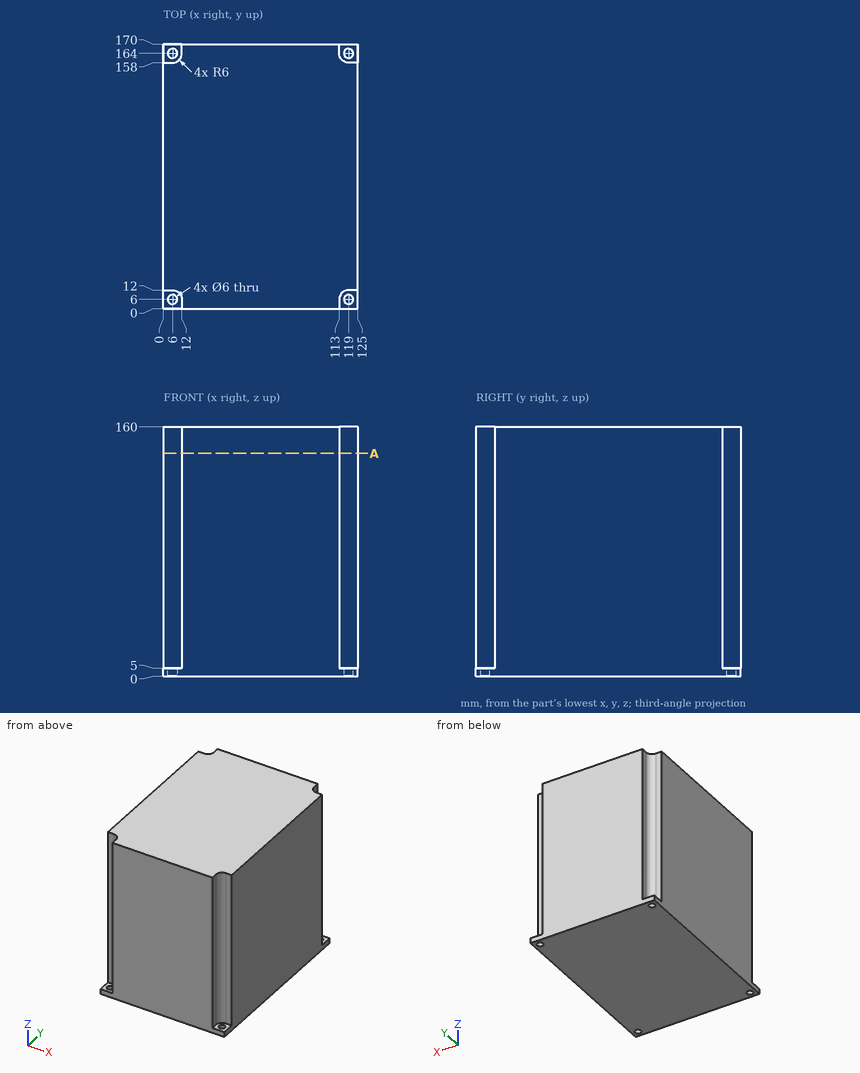
Geometry check sheet. Reference: drawing and pictorial views, mm from the part's lowest x, y, z. Give positions to 0.01 mm unless a question says otherwise; leave off trailing zeros. Write each loop counter-clockwise with the first axis right and the second up, starting at its lowest first coordinate (ties: lowest second). Pieces come first, ordered by that corner, then holes. Notation, with made-up numbers: M 11.25,70 L 45.25,70 A25 cw 45.25,98 Z; hole C 56.25,43.25 d10. An arc over 180 degrees is marked long. Answer as CSV lines item,"result". Start each with the question number.
Q1. Section check A-A, the plane z = 143. Record the cut outline in (x, y), then the cut area to 3 significant figures.
Q2. Go/stop test with flat-tipped pins: pin 1 (1.8 mm diameter, centred on y = 168, z = 118.5, fed in from -X); pin 2 (3 mm diameter, centred on x = 2.5, z = 54.5, fed in from -Y); pin 3 (1.8 mm diameter, centred on x = 121.5, z = 77.5, fed in from +Y); pin 4 (5 mm diameter, centred on x = 119, y = 164, fed in from -Z). Record where each tip stops, or that it passes through.
Q3. Material ranges on L1, parallel to Y at x = 119, z = 2; L2, parallel to X at y = 164, z = 3.95; L3, parallel to X at y = 8.5, z = 55, recorded low to high.
Geometry says:
1,outline,"M 0,12 L 6,12 A6 cw 12,6 L 12,0 L 113,0 L 113,6 A6 cw 119,12 L 125,12 L 125,158 L 119,158 A6 cw 113,164 L 113,170 L 12,170 L 12,164 A6 cw 6,158 L 0,158 Z"
1,area,"20,700 mm^2"
2,pin 1,"x = 12"
2,pin 2,"y = 12"
2,pin 3,"y = 158"
2,pin 4,"through"
3,L1,"0 to 3, 9 to 161, 167 to 170"
3,L2,"0 to 3, 9 to 116, 122 to 125"
3,L3,"11.45 to 113.55"
